Input: part model. Units: mm. Frame: model coordinates. Face numbers are marked on the shaded views. Round coordinates to 2 decimals unless told otherwise and drop trailing zeros. Order: outer loops, then holes, each group sorted by start corner. A loop starts at its lowest first (then second) coordinate and runs counter-clockwise, first axis right, second up.
Item 1: Mould query, pull axis Z, two halves, no side actions, for the marked faces 1, 2 and 3. Classes: released by +Z, released by -Z, zero draft, split by the parting line, or undercut.
Item 2: First-contact query: pin 1 (5 mm diameter, centred on y = 0, z = 4.5, fed in from -X); pin 2 (2 mm diameter, centred on x = 1, y = -2, fed in from +Z). Flat tips, straight axial feed; report the tip coordinate or a pass-through.
Item 3: Cut plane A-A on x = -0.3. Output: boundary loops of the cut face in (y, z), then the cut area to 3 significant figures.
Item 4: Cut plane C-C on y = 2. Give the number of separate pieces and of enclosed holes in the cut face, then the cut area to 3 significant figures.
Item 5: Line query: L1, parallel to Y at x = 0.45, z = 28; L2, parallel to Z at x = 1.35, y = 1; L3, parallel to Z at x = 0.95, y = -1.25. Output: solid intervals per line, ascending.
Item 6: Cut plane B-B on z = 26.5. Output: boundary loops of the cut face in (x, y).
```python
from build123d import *

# Parameters (mm, degrees)
CROQUIS1_R              = 2.75
SALIENTE_EXTRUIR4_DEPTH = 2
REDONDEO1_R             = 0.5


with BuildPart() as part:
    # Croquis1 → Saliente-Extruir4 (new, symmetric)
    with BuildSketch(Plane.YZ):
        with BuildLine():
            ThreePointArc((0, 32.5), (-3.181980515, 31.181980515), (-4.5, 28))
            Line((-4.5, 28), (-4.5, 15))
            Line((-4.5, 15), (-4.5, 9))
            Line((-4.5, 9), (-4.5, 4.5))
            ThreePointArc((-4.5, 4.5), (-3.181980515, 1.318019485), (0, 0))
            ThreePointArc((0, 0), (3.181980515, 1.318019485), (4.5, 4.5))
            Line((4.5, 4.5), (4.5, 9))
            Line((4.5, 9), (4.5, 15))
            Line((4.5, 15), (4.5, 28))
            ThreePointArc((4.5, 28), (3.181980515, 31.181980515), (0, 32.5))
        make_face()
        with Locations(Location((0, 4.5, 0), (0, 0, 270))):
            Circle(CROQUIS1_R, mode=Mode.SUBTRACT)
        with Locations(Location((0, 28, 0), (0, 0, 270))):
            Circle(CROQUIS1_R, mode=Mode.SUBTRACT)
    extrude(amount=SALIENTE_EXTRUIR4_DEPTH, both=True)

    # Redondeo1
    redondeo1_edges = [part.edges().sort_by_distance(p)[0] for p in [
        (-2, -4.5, 16.25),
        (2, -4.5, 16.25),
        (2, 0, 0),
        (2, 4.5, 16.25),
        (2, 0, 32.5),
        (-2, 0, 32.5),
        (-2, 4.5, 16.25),
        (-2, 0, 0),
    ]]
    fillet(redondeo1_edges, radius=REDONDEO1_R)


solid = part.part
```
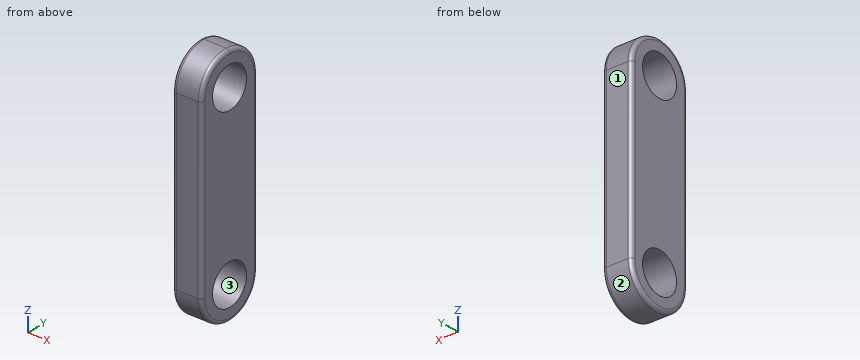
From the geometry:
1. face 1: zero draft
1. face 2: released by -Z
1. face 3: undercut
2. pin 1: passes through
2. pin 2: stops at z = 32.39
3. outline: (-4.5, 4.5) arc R4.5 ccw to (4.5, 4.5) - (4.5, 28) arc R4.5 ccw to (-4.5, 28) - close; hole circle Ø5.5 at (0, 4.5); hole circle Ø5.5 at (0, 28)
3. area: 228 mm2
4. separate pieces: 3
4. enclosed holes: 0
4. area: 95.8 mm2
5. L1: y = -4.5 to -2.75, 2.75 to 4.5
5. L2: z = 0.11 to 1.94, 7.06 to 25.44, 30.56 to 32.39
5. L3: z = 0.18 to 2.05, 6.95 to 25.55, 30.45 to 32.32
6. outline: (-2, -4) arc R0.5 ccw to (-1.5, -4.5) - (1.5, -4.5) arc R0.5 ccw to (2, -4) - (2, -2.3) - (-2, -2.3) - close; (-2, 2.3) - (2, 2.3) - (2, 4) arc R0.5 ccw to (1.5, 4.5) - (-1.5, 4.5) arc R0.5 ccw to (-2, 4) - close
